Input: dimensioned drawing with shaded views. Units: mm. Origin: part minimum x, y, z. A direction names the side the tool comes from. Coordinates: 2 decimals unless noted, no trailing zeros. Order: outer loops, then holes, each group sorted by start corner. A loop starts at its lowest first (then second) coordinate and runs counter-clockwise, first axis right, second up. Notation, with made-up numbers: (49.5, 43.5) - (70.5, 43.5) arc R23 cw to (70.5, 71.5) - close; hole circle Ø3 at (54, 10.25). An arc over 180 degrees is marked (long way). Answer as CSV lines item,"result". Start each with the question number.
Item 1: Section D-D (x = 40). Output: boundary loops of the cut face in (y, z), and give its area (3 significant figures).
Item 2: First-contact query: pin 1 (2.5 mm diameter, centred on x = 76, z = 4, fed in from +Y); pin 2 (4 mm diameter, centred on y = 21, z = 4, fed in from +X); pin 3 (4 mm diameter, centred on y = 14.5, z = 6, fed in from -X); pin 4 (5 mm diameter, centred on x = 68, y = 46.5, fed in from -Z). Flat tips, straight axial feed; report the tip coordinate or a pass-through.
Item 3: Section A-A (y = 13). Output: boundary loops of the cut face in (x, z).
Item 4: Section C-C (x = 76). Output: boundary loops of the cut face in (y, z).
Item 5: Material intervals for line 1 along X through (y, z) = (0.65, 4); line 2 along Z through (x, y) = (76, 1); line 3 along X through (y, z) = (15.5, 3.75), sorted ascending.
Item 6: Access query for the marked faces 4, 5, 6 and 7. Directions: +Z, -Z, +X, -X, +Y, -Y. A direction counts if a zero-diameter tool reaches every point of the face in a straight line with its end or side. Return the directions, or none.
Item 7: Section B-B (z = 4). Output: boundary loops of the cut face in (x, y).
Item 8: Draft query along X for the marked faces 1, 2 and 3. Return one class per face: +X half, -X half, draft (parallel to the pull), parting line (faces both ways), or undercut.
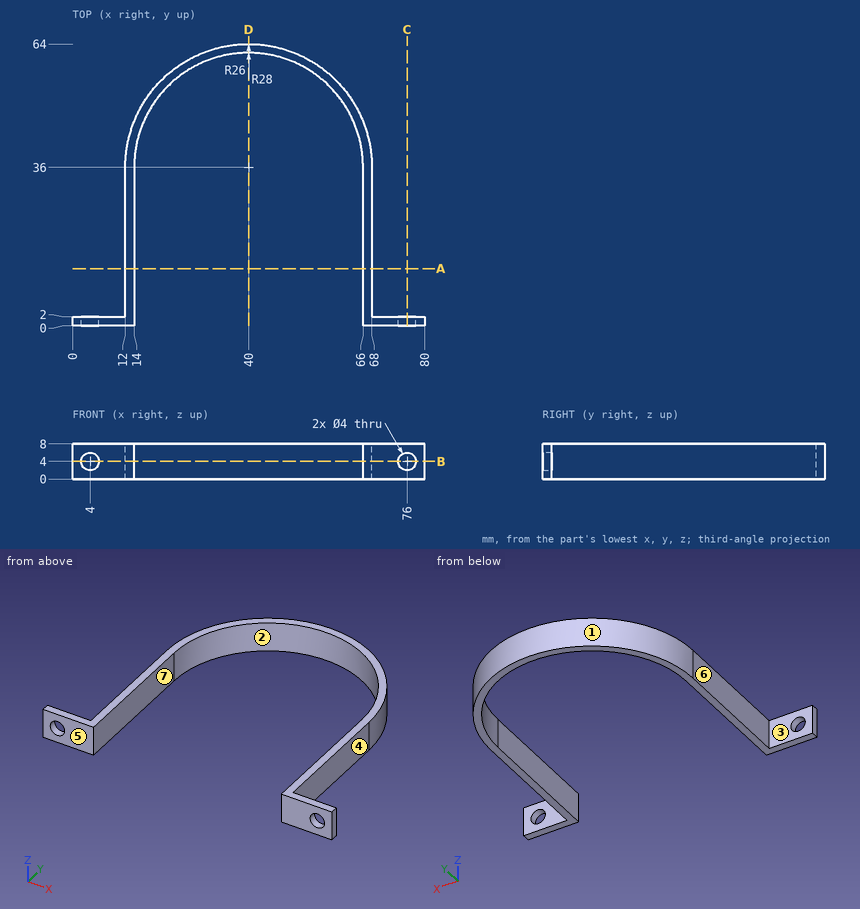
Determined:
1,outline,"(62, 0) - (64, 0) - (64, 8) - (62, 8) - close"
1,area,"16.0 mm^2"
2,pin 1,"passes through"
2,pin 2,"stops at x = 68"
2,pin 3,"stops at x = 12"
2,pin 4,"stops at z = 0"
3,outline,"(12, 0) - (14, 0) - (14, 8) - (12, 8) - close; (66, 0) - (68, 0) - (68, 8) - (66, 8) - close"
4,outline,"(0, 0) - (2, 0) - (2, 2) - (0, 2) - close; (0, 6) - (2, 6) - (2, 8) - (0, 8) - close"
5,line 1,"x = 0 to 2, 6 to 14, 66 to 74, 78 to 80"
5,line 2,"z = 0 to 2, 6 to 8"
5,line 3,"x = 12 to 14, 66 to 68"
6,face 4,"+Z, -Z, +X, +Y"
6,face 5,"+Z, -Z, +X, -X, -Y"
6,face 6,"+Z, -Z, -X, +Y"
6,face 7,"+Z, -Z, -Y"
7,outline,"(0, 0) - (2, 0) - (2, 2) - (0, 2) - close; (6, 0) - (14, 0) - (14, 36) arc R26 cw to (66, 36) - (66, 0) - (74, 0) - (74, 2) - (68, 2) - (68, 36) arc R28 ccw to (12, 36) - (12, 2) - (6, 2) - close; (78, 0) - (80, 0) - (80, 2) - (78, 2) - close"
8,face 1,"parting line"
8,face 2,"undercut"
8,face 3,"draft"
